Check sheet for the modelled part. Datum: model origin and axes. Units: mm. Face numbers are marked on the shaded views. A direction names the side the tool comes from. Coordinates: 2 decimals unless noted, no trailing zeros. Write each loop counter-clockwise with the first axis right and the second up, starting at its lowest first coordinate (ties: lowest second). Pieces come first, ordered by that corner, then holes. Notation, with made-up numbers: (58, 63.5) -> (77, 63.5) arc R27 cw to (77, 91.5) -> close; hole circle Ø11 at (3.5, 56). An arc over 180 degrees is marked (long way). Put each result on its own line as item: value.
```python
from build123d import *

# Parameters (mm, degrees)
F0_R      = 6
F2_DEPTH  = 3
F3_W      = 20
F3_H      = 8
F4_DEPTH  = 14
F1_R      = 6
F4_FACE_W = 20
F4_FACE_H = 8
F5_DEPTH  = 3


with BuildPart() as f2:
    # F0 (on Front) → F2 (new body)
    with BuildSketch(Plane.XZ):
        with BuildLine():
            ThreePointArc((-12, 0), (-20, -8), (-12, -16))
            Line((-12, -16), (20, -16))
            ThreePointArc((20, -16), (28, -8), (20, 0))
            Line((20, 0), (20, 8))
            Line((20, 8), (0, 8))
            Line((0, 8), (0, 0))
            Line((0, 0), (-12, 0))
        make_face()
        with Locations((-12, -8)):
            Circle(F0_R, mode=Mode.SUBTRACT)
        with Locations((20, -8)):
            Circle(F0_R, mode=Mode.SUBTRACT)
    extrude(amount=F2_DEPTH)

    # F3 (on Front) → F4 (join)
    with BuildSketch(Plane.XZ):
        with Locations((10, 4)):
            Rectangle(F3_W, F3_H)
    extrude(amount=F4_DEPTH)

    # F1 (on Front) + F4_face (on face) → F5 (join)
    with BuildSketch(Plane.XZ):
        with BuildLine():
            Line((0, 8), (0, 0))
            Line((0, 0), (-12, 0))
            ThreePointArc((-12, 0), (-20, -8), (-12, -16))
            Line((-12, -16), (20, -16))
            ThreePointArc((20, -16), (28, -8), (20, 0))
            Line((20, 0), (20, 8))
            Line((20, 8), (0, 8))
        make_face()
        with Locations((-12, -8)):
            Circle(F1_R, mode=Mode.SUBTRACT)
        with Locations((20, -8)):
            Circle(F1_R, mode=Mode.SUBTRACT)
    with BuildSketch(Plane(origin=(10, -14, 4), x_dir=(1, 0, 0), z_dir=(0, -1, 0))):
        Rectangle(F4_FACE_W, F4_FACE_H)
    extrude(amount=-F5_DEPTH)


solid = f2.part
```
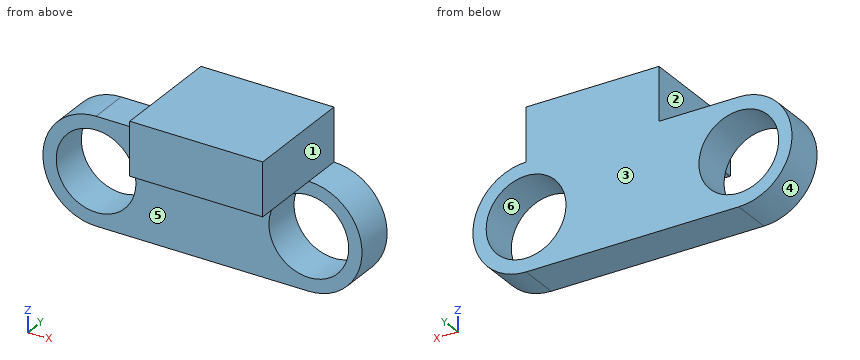
Q1. Cross-section at B-B (y = -2). Record the cut outline in (x, z).
Recorded:
outline: (-12, -16) -> (20, -16) arc R8 ccw to (20, 0) -> (20, 8) -> (0, 8) -> (0, 0) -> (-12, 0) arc R8 ccw to start; hole circle Ø12 at (-12, -8); hole circle Ø12 at (20, -8)
Q2. Cross-section at D-D (x = 9). Record the cut outline in (y, z).
Recorded:
outline: (-14, 0) -> (-3, 0) -> (-3, -16) -> (3, -16) -> (3, 8) -> (-14, 8) -> close
Q3. Cross-section at A-A (z = -8). Record the cut outline in (x, y).
Recorded:
outline: (-20, -3) -> (-18, -3) -> (-18, 3) -> (-20, 3) -> close; (-6, -3) -> (14, -3) -> (14, 3) -> (-6, 3) -> close; (26, -3) -> (28, -3) -> (28, 3) -> (26, 3) -> close
Q4. Cross-section at C-C (x = 25.5). Record the cut outline in (y, z).
Recorded:
outline: (-3, -13.81) -> (3, -13.81) -> (3, -10.4) -> (-3, -10.4) -> close; (-3, -5.6) -> (3, -5.6) -> (3, -2.19) -> (-3, -2.19) -> close
Q5. Tool access check on the marked faces 1, 2 and 3. Record the directions out of +Z, -Z, +X, -X, +Y, -Y that give a thin tool (end or side, any length) a straight path to the whole face; none if there is none.
Recorded:
face 1: +Z, +X, +Y, -Y
face 2: +Z, -X, +Y, -Y
face 3: +Z, -Z, +X, -X, +Y
Q6. Material ranges on line 1 along Z through (x, y) = (-12, 0.3); line 2 along X through (y, z) = (-11.5, 3.75); line 3 along Y through (x, z) = (-1, -14.5), recorded low to high.
Recorded:
line 1: z = -16 to -14, -2 to 0
line 2: x = 0 to 20
line 3: y = -3 to 3
Q7. Depth check by flat-ended pin: P1, Ø5, axis at x = -6, y = 1.5, coming from the +Z side; P2, Ø2, axis at y = -5, z = -4.5, coming from the +X side; P3, Ø6.5, axis at y = -9, z = 6, coming from the -X side; P4, Ø5, axis at x = 12.5, z = -10, coming from the -Y side. Enter the tip coordinate at first touch or a pass-through.
Recorded:
P1: stops at z = 0
P2: passes through
P3: stops at x = 0
P4: stops at y = -3
Q8. Mould release check, pull along X, two halves, no side actions. Record for the marked faces 4, 5 and 6: released by +X, released by -X, zero draft, split by the parting line, or undercut.
Recorded:
face 4: released by -X
face 5: zero draft
face 6: undercut
